from build123d import *

# Parameters (mm, degrees)
F1_DEPTH = 2
F2_W     = 1.2
F2_H     = 25
F3_DEPTH = 0.4
F4_W     = 1.2
F4_H     = 25
F5_DEPTH = 0.4


with BuildPart() as f1:
    # F0 (on Top) → F1 (new body)
    with BuildSketch(Plane.XY):
        with BuildLine():
            Line((0, 25), (0, 0))
            Line((0, 0), (70, 0))
            Line((70, 0), (70, 0.351166))
            ThreePointArc((70, 0.351166), (68.327306, 4.507417), (64.24186, 6.34629))
            ThreePointArc((64.24186, 6.34629), (34.416213, 11.508745), (6.947288, 24.224025))
            ThreePointArc((6.947288, 24.224025), (5.664732, 24.802089), (4.271916, 25))
            Line((4.271916, 25), (0, 25))
        make_face()
        Polygon((12.798805, 15.11953), (17.467075, 15.942672), (15.845802, 11.488261), (18.750836, 8.026177), (14.300066, 7.241386), (12.678793, 2.786975), (9.631796, 6.418244), (4.963527, 5.595102), (6.5848, 10.049513), (3.679766, 13.511597), (8.130536, 14.296388), (9.751809, 18.750799), align=None, mode=Mode.SUBTRACT)
        Polygon((27.314466, 9.476318), (29.033361, 11.195212), (29.66252, 8.847159), (31.797244, 8.275161), (30.234517, 6.712435), (30.863677, 4.364381), (28.515623, 4.99354), (26.796728, 3.274646), (26.167569, 5.622699), (24.032845, 6.194697), (25.595572, 7.757423), (24.966413, 10.105477), align=None, mode=Mode.SUBTRACT)
    extrude(amount=F1_DEPTH)

    # F2 (on face) → F3 (cut)
    with BuildSketch(Plane.XY.offset(2)):
        with Locations((2.4, 12.5)):
            Rectangle(F2_W, F2_H)
    extrude(amount=-F3_DEPTH, mode=Mode.SUBTRACT)

    # F4 (on face) → F5 (cut)
    with BuildSketch(Plane(origin=(0, 0, 0), x_dir=(1, 0, 0), z_dir=(0, 0, -1))):
        with Locations((2.4, -12.5)):
            Rectangle(F4_W, F4_H)
    extrude(amount=-F5_DEPTH, mode=Mode.SUBTRACT)


solid = f1.part
Geometry: final body of the model. Coordinates: model frame, mm. A direction names the side the tool comes from. Give positions to 0.01 mm unless a question says otherwise; leave off trailing zeros. Write each loop counter-clockwise with the first axis right and the second up, starting at its lowest first coordinate (ties: lowest second). Pieces come first, ordered by that corner, then holes.
(1) Cut plane A-A, the plane z = 1. Give the number of separate pieces and of enclosed holes in the cut face, then the cut area to 3 significant figures.
(2) First-contact query: P1, Ø10, axis at x = 38.5, y = 4, coming from the -Z side; P2, Ø0.6, axis at x = 2.5, y = 15.5, coming from the +Z side. Flat tips, straight axial feed; report the tip coordinate or a pass-through.
(3) Cut plane C-C, the plane y = 23. Return loops of the section in (x, z), then the cut area to 3 significant figures.
(4) Ray query, line 1 (X direction, y = 18.25, z = 1.8); line 2 (X direction, y = 3.5, z = 0.95); line 3 (X direction, y = 22.25, z = 0.35). Return the intervals inside material, ascending.
(5) Access query for faces 1 (the flat face through (2, 13, 1.6)), 2 (the flat face through (8.93, 16.49, 0.99)), 3 (the cylindrical face through (5.684, 24.797, 0.986)), 4 (the flat face through (2, 12, 0.4)). Directions: +Z, -Z, +X, -X, +Y, -Y. A direction counts if a zero-diameter tool reaches every point of the face in a straight line with its end or side. Return the directions, or none.
(6) Mould query, pull axis X, two halves, no side actions, for faces 5 (the flat face through (1, 13, 0)), 6 (the cylindrical face through (68.37, 4.46, 0.99)), 7 (the flat face through (5.874, 13.898, 0.986)). Classes: released by +X, released by -X, zero draft, split by the parting line, or undercut.
(7) Cut plane B-B, the plane x = 13.5. Return loops of the section in (y, z).
(8) Cut plane D-D, the plane x = 44. Return loops of the section in (y, z), then the cut area to 3 significant figures.
Values follow:
1. separate pieces: 1
1. enclosed holes: 2
1. area: 777 mm2
2. P1: stops at z = 0
2. P2: stops at z = 1.6
3. outline: (0, 0) - (1.8, 0) - (1.8, 0.4) - (3, 0.4) - (3, 0) - (8.92, 0) - (8.92, 2) - (3, 2) - (3, 1.6) - (1.8, 1.6) - (1.8, 2) - (0, 2) - close
3. area: 16.9 mm2
4. line 1: x = 0 to 1.8, 3 to 9.57, 10.17 to 17.58
4. line 2: x = 0 to 12.08, 12.94 to 26.74, 27.02 to 69.11
4. line 3: x = 0 to 1.8, 3 to 10.18
5. face 1: +Z, +Y, -Y
5. face 2: +Z, -Z
5. face 3: +Z, -Z, +X, +Y
5. face 4: -Z, +Y, -Y
6. face 5: zero draft
6. face 6: released by +X
6. face 7: undercut
7. outline: (0, 0) - (5.04, 0) - (5.04, 2) - (0, 2) - close; (15.24, 0) - (20.37, 0) - (20.37, 2) - (15.24, 2) - close
8. outline: (0, 0) - (8.96, 0) - (8.96, 2) - (0, 2) - close
8. area: 17.9 mm2
